Design review of the part built by this model. Coordinates are the model's own, in mm. A direction names the side the tool comes from. Round coordinates to 2 decimals unless told otherwise and drop trailing zeros. Write each loop counter-clockwise with the first axis right and the second up, starting at its lowest first coordinate (ties: lowest second). Pieces come first, ordered by that corner, then holes. Notation, with made-up numbers: M -38,-16 L 3,-16 A6 cw 3,-9 Z; hole C -25.5,50 d6. An arc over 180 degrees is marked long. Use CSV: the item, a comma, the result in double quotes.
from build123d import *

# Parameters (mm, degrees)
SKETCH_1_R      = 1.5
EXTRUDE_1_DEPTH = 3


with BuildPart() as part:
    # 草图1 → 凸台-拉伸1 (new body)
    with BuildSketch(Plane(origin=(0, 0, 0), x_dir=(-1, 0, 0), z_dir=(0, 0, -1))):
        with BuildLine():
            Line((-108.521309774, 0), (16.478690226, 0))
            ThreePointArc((16.478690226, 0), (23.549758037, 2.928932188), (26.478690226, 10))
            Line((26.478690226, 10), (26.478690226, 84.99928))
            ThreePointArc((26.478690226, 84.99928), (23.549758037, 92.070347812), (16.478690226, 94.99928))
            Line((16.478690226, 94.99928), (-108.521309774, 94.99928))
            ThreePointArc((-108.521309774, 94.99928), (-115.592377586, 92.070347812), (-118.521309774, 84.99928))
            Line((-118.521309774, 84.99928), (-118.521309774, 10))
            ThreePointArc((-118.521309774, 10), (-115.592377586, 2.928932188), (-108.521309774, 0))
        make_face()
        with Locations(Location((15.978690226, 67.81454533, 0), (0, 0, 180))):
            Circle(SKETCH_1_R, mode=Mode.SUBTRACT)
        with Locations(Location((-32.220309774, 66.51524533, 0), (0, 0, 180))):
            Circle(SKETCH_1_R, mode=Mode.SUBTRACT)
        with Locations(Location((10.878690226, 15.71504533, 0), (0, 0, 180))):
            Circle(SKETCH_1_R, mode=Mode.SUBTRACT)
        with Locations(Location((-54.521309774, 69.37594533, 0), (0, 0, 180))):
            Circle(SKETCH_1_R, mode=Mode.SUBTRACT)
        with Locations(Location((-98.520309774, 69.37594533, 0), (0, 0, 180))):
            Circle(SKETCH_1_R, mode=Mode.SUBTRACT)
        with Locations(Location((-98.520309774, 25.37514533, 0), (0, 0, 180))):
            Circle(SKETCH_1_R, mode=Mode.SUBTRACT)
        with Locations(Location((-54.521309774, 25.37514533, 0), (0, 0, 180))):
            Circle(SKETCH_1_R, mode=Mode.SUBTRACT)
        with Locations(Location((-17.021309774, 15.71504533, 0), (0, 0, 180))):
            Circle(SKETCH_1_R, mode=Mode.SUBTRACT)
        with BuildLine():
            Line((-109.719554185, 49.655521805), (-78.625612362, 80.786563559))
            ThreePointArc((-78.625612362, 80.786563559), (-76.504816284, 81.666507838), (-74.382972429, 80.789093116))
            Line((-74.382972429, 80.789093116), (-43.251668672, 49.694889603))
            ThreePointArc((-43.251668672, 49.694889603), (-42.371724394, 47.574093524), (-43.249139115, 45.452249669))
            Line((-43.249139115, 45.452249669), (-74.343080939, 14.321207916))
            ThreePointArc((-74.343080939, 14.321207916), (-76.463877017, 13.441263637), (-78.585720872, 14.318678358))
            Line((-78.585720872, 14.318678358), (-109.717024628, 45.412881872))
            ThreePointArc((-109.717024628, 45.412881872), (-110.596968907, 47.53367795), (-109.719554185, 49.655521805))
        make_face(mode=Mode.SUBTRACT)
    extrude(amount=-EXTRUDE_1_DEPTH)


solid = part.part
1) Add section A-A on y = 44. Write out the cut boundary in (x, z), then the cut area to 3 significant figures.
Answers:
outline,"M -26.48,0 L 44.7,0 L 44.7,3 L -26.48,3 Z; M 108.3,0 L 118.52,0 L 118.52,3 L 108.3,3 Z"
area,"244 mm²"
2) Machinability: for faces 1 (the face through (115.67, 3.01, 1.48)), 2 (the face through (76.538, 81.666, 1.479)), which of the approach directions +Z, -Z, +X, -X, +Y, -Y give a long, thin tool a straight path to every point of the face, cutting with its end or side? Answer none if there is none.
Answers:
face 1,"+Z, -Z, +X, -Y"
face 2,"+Z, -Z"
3) For pin 1 Ø2.5 at (x, y) = (-10.88, 15.72) entering from +Z, flat-tipped, find the tip position at first contact; note if it passes through.
Answers:
pin 1,"through"
4) Add section B-B on x = 47.5. Write out the cut boundary in (y, z), then the cut area to 3 significant figures.
Answers:
outline,"M 0,0 L 41.2,0 L 41.2,3 L 0,3 Z; M 53.94,0 L 95,0 L 95,3 L 53.94,3 Z"
area,"247 mm²"
5) Add section C-C on z = 2.15. Give the number of separate pieces and of enclosed holes in the cut face, then the cut area to 3 significant figures.
Answers:
separate pieces,"1"
enclosed holes,"9"
area,"11,100 mm²"
6) Wall thickness on line 1 along X through (y, z) = (26, 1.55); line 2 along X through (y, z) = (47.5, 2.75); line 3 along Y through (x, z) = (51.5, 2.2): over which ranges is each line inside the solid? List them lowest first. Write a range as [from, to].
Answers:
line 1,"[-26.48, 53.16], [55.88, 62.68], [90.28, 97.16], [99.88, 118.52]"
line 2,"[-26.48, 42.37], [110.6, 118.52]"
line 3,"[0, 37.19], [57.93, 95]"
